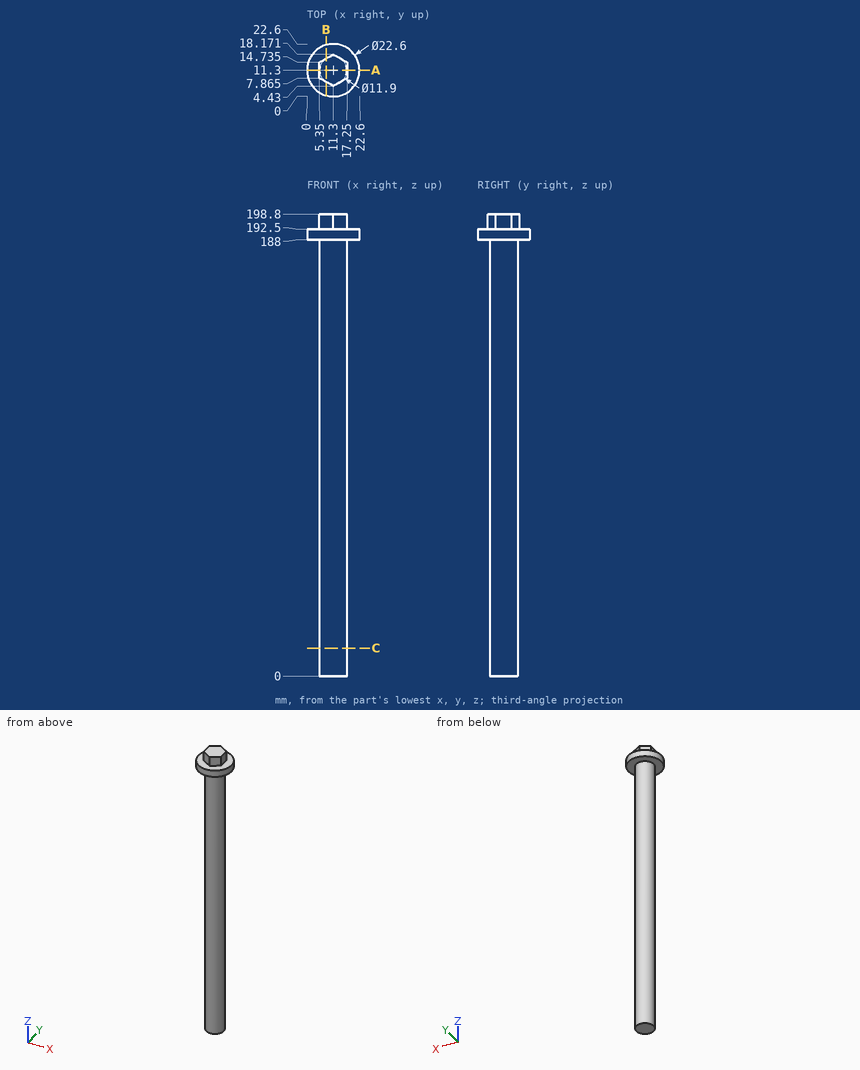
Geometry check sheet. Reference: drawing and pictorial views, mm from the part's lowest x, y, z. Give positions to 0.01 mm unless a question says otherwise; leave off trailing zeros. Loops run counter-clockwise (first coordinate to the right, second up) from the corner with the lowest first, then second, coordinate; pieces in that order, holes last.
1. Section check A-A, the plane y = 11.3. Enter the section's corners in (x, z), then the cut area to 3 significant figures.
2. Go/stop test with flat-tipped pins: pin 1 Ø5 at (y, z) = (12, 195.5) entering from +X; pin 2 Ø5 at (x, z) = (12, 132.5) entering from -Y; pin 3 Ø6 at (y, z) = (4.5, 51.5) entering from +X. Record where each tip stops, or that it passes through.
3. Section check B-B, the plane x = 8.25. Enter the section's corners in (y, z), then the cut area to 3 significant figures.
4. Thickness scan on line 1 (Z direction, x = 8, y = 17.5); line 2 (X direction, y = 7.5, z = 107.5); line 3 (Y direction, x = 16.75, z = 71) (1 decimal). Record the ranges inside material, lowest first.
5. Section check C-C, the plane z = 12. Enter the section's corners in (x, y), then the cut area to 3 significant figures.
Geometry says:
1. outline: (0, 188) - (5.35, 188) - (5.35, 0) - (17.25, 0) - (17.25, 188) - (22.6, 188) - (22.6, 192.5) - (17.25, 192.5) - (17.25, 198.8) - (5.35, 198.8) - (5.35, 192.5) - (0, 192.5) - close
1. area: 2,410 mm2
2. pin 1: stops at x = 17.25
2. pin 2: stops at y = 5.35
2. pin 3: stops at x = 15.88
3. outline: (0.42, 188) - (6.19, 188) - (6.19, 0) - (16.41, 0) - (16.41, 188) - (22.18, 188) - (22.18, 192.5) - (16.41, 192.5) - (16.41, 198.8) - (6.19, 198.8) - (6.19, 192.5) - (0.42, 192.5) - close
3. area: 2,080 mm2
4. line 1: z = 188 to 192.5
4. line 2: x = 6.72 to 15.88
4. line 3: y = 8.9 to 13.7
5. outline: circle Ø11.9 at (11.3, 11.3)
5. area: 111 mm2
